```python
from build123d import *

# Parameters (mm, degrees)
SKETCH1_W           = 16.75
SKETCH1_H           = 23.5
BOSS_EXTRUDE1_DEPTH = 1.2
SKETCH3_R           = 0.75
BOSS_EXTRUDE2_DEPTH = 5.2
SKETCH5_W           = 16.75
SKETCH5_H           = 23.5
SKETCH5_W_2         = 16.15
SKETCH5_H_2         = 22.9
BOSS_EXTRUDE3_DEPTH = 7
SKETCH7_W           = 2.1
SKETCH7_H           = 15.24
BOSS_EXTRUDE5_DEPTH = 3.8
FILLET4_R           = 0.3


with BuildPart() as part:
    # Sketch1 → Boss-Extrude1 (new body)
    with BuildSketch(Plane(origin=(0, 0, 0), x_dir=(1, 0, 0), z_dir=(0, 1, 0))):
        with Locations((8.375, -11.75)):
            Rectangle(SKETCH1_W, SKETCH1_H)
    extrude(amount=BOSS_EXTRUDE1_DEPTH)

    # Sketch3 → Boss-Extrude2 (add)
    with BuildSketch(Plane(origin=(0, 1.2, 0), x_dir=(1, 0, 0), z_dir=(0, 1, 0))):
        with Locations(Location((2.3, -2.268544265, 0), (0, 0, 270))):
            Circle(SKETCH3_R)
        with Locations(Location((2.3, -21.2, 0), (0, 0, 270))):
            Circle(SKETCH3_R)
        with Locations(Location((14.45, -21.2, 0), (0, 0, 270))):
            Circle(SKETCH3_R)
        with Locations(Location((14.45, -2.3, 0), (0, 0, 270))):
            Circle(SKETCH3_R)
    extrude(amount=BOSS_EXTRUDE2_DEPTH)

    # Sketch5 → Boss-Extrude3 (add)
    with BuildSketch(Plane(origin=(0, 1.2, 0), x_dir=(1, 0, 0), z_dir=(0, 1, 0))):
        with Locations((8.375, -11.75)):
            Rectangle(SKETCH5_W, SKETCH5_H)
        with Locations((8.375, -11.75)):
            Rectangle(SKETCH5_W_2, SKETCH5_H_2, mode=Mode.SUBTRACT)
    extrude(amount=BOSS_EXTRUDE3_DEPTH)

    # Sketch7 → Boss-Extrude5 (add)
    with BuildSketch(Plane(origin=(0, 1.2, 0), x_dir=(1, 0, 0), z_dir=(0, 1, 0))):
        Polygon((2.45, -3.63), (4.55, -3.63), (4.75, -3.63), (4.75, -19.27), (2.25, -19.27), (2.25, -3.63), align=None)
        with Locations((3.5, -11.45)):
            Rectangle(SKETCH7_W, SKETCH7_H, mode=Mode.SUBTRACT)
    extrude(amount=BOSS_EXTRUDE5_DEPTH)

    # Fillet4
    fillet4_edges = [part.edges().sort_by_distance(p)[0] for p in [
        (0, 8.2, 11.75),
        (8.375, 8.2, 23.5),
        (16.75, 8.2, 11.75),
        (8.375, 8.2, 0),
        (8.375, 0, 0),
        (16.75, 0, 11.75),
        (8.375, 0, 23.5),
        (0, 0, 11.75),
        (0, 4.1, 0),
        (16.75, 4.1, 0),
        (16.75, 4.1, 23.5),
        (0, 4.1, 23.5),
    ]]
    fillet(fillet4_edges, radius=FILLET4_R - 0.0001)  # a hair under: the kernel refuses the full size


solid = part.part
```
Could you check a few things on this model? Use its own coordinates, in mm. Give positions to 0.01 mm unless a question says otherwise; leave off trailing zeros. Order: outer loops, then holes, each group sorted by start corner. A loop starts at its lowest first (then second) coordinate and runs counter-clockwise, first axis right, second up.
Q1. We'd pull the mould along X, two halves only. Please class faces 1 (the flat face through (8, 0, 12)), 2 (the cylindrical face through (2.33, 3.76, 1.52)): +X half, -X half, draft (parallel to the pull), parting line (faces both ways), or undercut.
Q2. If I drill on line 1 along X through (y, z) = (4.25, 17); line 2 along Z through (x, y) = (4.5, 4.5); line 3 along Z through (x, y) = (13.75, 7.75), over which ranges is the centre line in solid material (lowest first)?
Q3. Suppose I cut it at B-B, the plane y = 7.5. Write out the boundary of the cut face in (x, z), and give its area (3 significant figures).
Q4. I'm going to push flat-ended pins straight in: P1, Ø2, axis at x = 12.5, z = 15.5, coming from the +Y side; P2, Ø1.2, axis at x = 2.5, z = 21, coming from the +Y side. Where does each tip first touch, or does it pass through?
Q5. Suppose I cut it at A-A, the plane y = 2.75. Write out the boundary of the cut face in (x, z), and give its area (3 significant figures).
Solution:
1. face 1: draft
1. face 2: undercut
2. line 1: x = 0 to 0.3, 2.25 to 2.45, 4.55 to 4.75, 16.45 to 16.75
2. line 2: z = 0 to 0.3, 3.63 to 3.83, 19.07 to 19.27, 23.2 to 23.5
2. line 3: z = 0 to 0.3, 23.2 to 23.5
3. outline: (0, 0.3) arc R0.3 ccw to (0.3, 0) - (16.45, 0) arc R0.3 ccw to (16.75, 0.3) - (16.75, 23.2) arc R0.3 ccw to (16.45, 23.5) - (0.3, 23.5) arc R0.3 ccw to (0, 23.2) - close; hole (0.3, 0.3) - (16.45, 0.3) - (16.45, 23.2) - (0.3, 23.2) - close
3. area: 23.7 mm2
4. P1: stops at y = 1.2
4. P2: stops at y = 6.4
5. outline: (0, 0.3) arc R0.3 ccw to (0.3, 0) - (16.45, 0) arc R0.3 ccw to (16.75, 0.3) - (16.75, 23.2) arc R0.3 ccw to (16.45, 23.5) - (0.3, 23.5) arc R0.3 ccw to (0, 23.2) - close; circle Ø1.5 at (2.3, 2.27); circle Ø1.5 at (2.3, 21.2); (2.25, 3.63) - (4.75, 3.63) - (4.75, 19.27) - (2.25, 19.27) - close; circle Ø1.5 at (14.45, 2.3); circle Ø1.5 at (14.45, 21.2); hole (0.3, 0.3) - (16.45, 0.3) - (16.45, 23.2) - (0.3, 23.2) - close; hole (2.45, 3.83) - (4.55, 3.83) - (4.55, 19.07) - (2.45, 19.07) - close
5. area: 37.9 mm2
